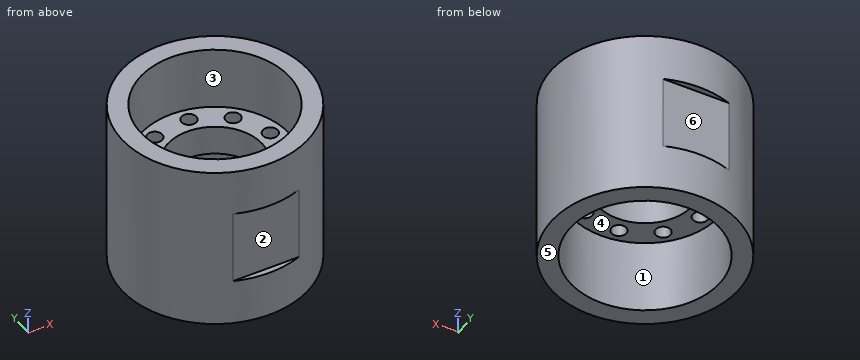
```python
from build123d import *

# Parameters (mm, degrees)
SKETCH1_R           = 25
BOSS_EXTRUDE1_DEPTH = 45
SKETCH2_R           = 20
CUT_EXTRUDE1_DEPTH  = 17
SKETCH3_R           = 12.7
CUT_EXTRUDE2_DEPTH  = 18
SKETCH4_R           = 2
CUT_EXTRUDE3_DEPTH  = 46.099889135
CIRPATTERN1_COUNT   = 10
CUT_EXTRUDE4_START  = -20
SKETCH5_R           = 20
CUT_EXTRUDE4_DEPTH  = 20
CUT_EXTRUDE8_DEPTH  = 10


with BuildPart() as part:
    # Sketch1 → Boss-Extrude1 (new body)
    with BuildSketch(Plane.XY):
        with Locations(Location((0, 0, 0), (0, 0, 180))):
            Circle(SKETCH1_R)
    extrude(amount=BOSS_EXTRUDE1_DEPTH)

    # Sketch2 → Cut-Extrude1 (cut)
    with BuildSketch(Plane.XY.offset(45)):
        Circle(SKETCH2_R)
    extrude(amount=-CUT_EXTRUDE1_DEPTH, mode=Mode.SUBTRACT)

    # Sketch3 → Cut-Extrude2 (cut)
    with BuildSketch(Plane.XY.offset(28)):
        Circle(SKETCH3_R)
    extrude(amount=-CUT_EXTRUDE2_DEPTH, mode=Mode.SUBTRACT)

    # Sketch4 → Cut-Extrude3 (cut, through all)
    with BuildSketch(Plane.XY.offset(28)):
        with Locations((-7.552723676, 14.669913602)):
            Circle(SKETCH4_R)
    cut_extrude3 = extrude(amount=-CUT_EXTRUDE3_DEPTH, mode=Mode.SUBTRACT)

    # CirPattern1: Cut-Extrude3 ×10 about axis
    cirpattern1_axis = Axis((0, 0, 0), (0, 0, 1))
    for i in range(1, CIRPATTERN1_COUNT):
        add(cut_extrude3.rotate(cirpattern1_axis, i * 360 / CIRPATTERN1_COUNT), mode=Mode.SUBTRACT)

    # Sketch5 → Cut-Extrude4 (cut)
    with BuildSketch(Plane(origin=(0, 0, 0), x_dir=(-1, 0, 0), z_dir=(0, 0, -1)).offset(CUT_EXTRUDE4_START)):
        with Locations(Location((0, 0, 0), (0, 0, 180))):
            Circle(SKETCH5_R)
    extrude(amount=CUT_EXTRUDE4_DEPTH, mode=Mode.SUBTRACT)

    # Sketch8 → Cut-Extrude8 (cut, symmetric)
    with BuildSketch(Plane.XY.offset(22.5)):
        with BuildLine():
            Line((-8.8, 23.4), (8.8, 23.4))
            ThreePointArc((8.8, 23.4), (0, 25), (-8.8, 23.4))
        make_face()
        with BuildLine():
            Line((-8.8, -23.4), (8.8, -23.4))
            ThreePointArc((8.8, -23.4), (0, -25), (-8.8, -23.4))
        make_face()
    extrude(amount=CUT_EXTRUDE8_DEPTH, both=True, mode=Mode.SUBTRACT)


solid = part.part
```
Could you check a few things on this model? Use its own coordinates, in mm. Face numbers are marked on the shaded views. A direction names the side the tool comes from. Round coordinates to 2 decimals unless told otherwise and drop trailing zeros. Loops run counter-clockwise (first coordinate to the right, second up) from the corner with the lowest first, then second, coordinate; pieces in that order, holes last.
Q1. I want a section at C-C (x = -11.5). Write out the boundary of the cut face in (y, z), and give its area (3 significant figures).
Q2. I want a section at D-D (x = -21). Write out the boundary of the cut face in (y, z).
Q3. I want a section at B-B (y = 11). Write out the boundary of the cut face in (x, z).
Q4. Thinking about a two-plate mould opening in Y: for the marked faces 4, 5 and 6, which applies, pulls with the +Y half, pulls with the -Y half, needs draft (parallel to the pull), parting line crosses it, or undercut?
Q5. For P1, Ø4, axis at x = -1.5, z = 16.5, coming from the +Y side; P2, Ø6, axis at x = 8.5, z = 39, coming from the +Y side; P3, Ø4.5, axis at x = -7.55, y = 14.67, coming from the -Z side; P4, Ø1.8, axis at x = 1.5, y = -24, coming from the -Z side, each with a flat end and sliding along its axis, tell me the tip position at first contact or that it passes through.
Q6. Please list where these lines run through material, in increasing order: L1, parallel to Y at x = -6.5, z = 24; L2, parallel to X at y = 15, z = 21; L3, parallel to Z at x = -5, y = 23.5.
Q7. I want a section at A-A (z = 29). Write out the boundary of the cut face in (x, y).
Q8. On a 3-axis mill with a long thin cutter (end or side, diameter ignored), from which of +Z, -Z, +X, -X, +Y, -Y can I reach the whole of each face in a straight line? I mean the marked faces 1, 2 and 3. Say none if no direction works.
Answer below:
1. outline: (-22.2, 0) - (-16.36, 0) - (-16.36, 20) - (-13.71, 20) - (-13.71, 28) - (-16.36, 28) - (-16.36, 45) - (-22.2, 45) - close; (-9.72, 20) - (-5.39, 20) - (-5.39, 28) - (-9.72, 28) - close; (5.39, 20) - (16.36, 20) - (16.36, 0) - (22.2, 0) - (22.2, 45) - (16.36, 45) - (16.36, 28) - (5.39, 28) - close
1. area: 669 mm2
2. outline: (-13.56, 0) - (13.56, 0) - (13.56, 45) - (-13.56, 45) - close
3. outline: (-22.45, 0) - (-16.7, 0) - (-16.7, 20) - (-6.35, 20) - (-6.35, 28) - (-16.7, 28) - (-16.7, 45) - (-22.45, 45) - close; (6.35, 20) - (9.75, 20) - (9.75, 28) - (6.35, 28) - close; (13.49, 20) - (16.7, 20) - (16.7, 0) - (22.45, 0) - (22.45, 45) - (16.7, 45) - (16.7, 28) - (13.49, 28) - close
4. face 4: undercut
4. face 5: needs draft
4. face 6: pulls with the +Y half
5. P1: stops at y = 23.4
5. P2: stops at y = 24.39
5. P3: stops at z = 20
5. P4: stops at z = 0
6. L1: y = -23.4 to -10.91, 10.91 to 12.97, 16.37 to 23.4
6. L2: x = -20 to -9.53, -5.58 to 1, 4.03 to 20
6. L3: z = 0 to 12.5, 32.5 to 45
7. outline: (-8.8, -23.4) - (8.8, -23.4) arc R25 ccw to (8.8, 23.4) - (-8.8, 23.4) arc R25 ccw to start; hole circle Ø40 at (0, 0)
8. face 1: -Z
8. face 2: +X, -X, -Y
8. face 3: +Z
